Geometry: final body of the model. Coordinates: model frame, mm. Face numbers are marked on the shaded views. Round coordinates to 2 decimals unless told otherwise and drop trailing zeros. Order: outer loops, then holes, each group sorted by start corner. A loop starts at its lowest first (then second) coordinate and runs counter-clockwise, first axis right, second up. Notation, with made-up numbers: (37.25, 7.25) - (49.25, 7.25) arc R19 ccw to (49.25, 39.25) - close; hole circle Ø4 at (42.25, -40). An arc over 180 degrees is marked (long way). Put each result on its own line as item: value. Start each with the question number.
(1) Section C-C (y = -1886.5). Output: boundary loops of the cut face in (x, z), and give its area (3 significant figures).
(2) Pin query (flat end, axial travel): P1, Ø6, axis at x = -21.5, y = -366, coming from the +Z side; P2, Ø2, axis at y = -1765.5, z = 63.5, coming from the -X side; P3, Ø1, axis at y = -359, z = -63.5, coming from the -X side. Return the tip coordinate at first contact, or that it passes through.
(3) Pull-direction query (Y, two-part tool) for the marked faces 1, 2 and 3; classes: released by +Y, released by -Y, zero draft, split by the parting line, or undercut.
(4) Section B-B (z = -42.5). Output: boundary loops of the cut face in (x, y).
(5) Material intervals for L1, parallel to Z at x = -75, y = -2038.5; L2, parallel to Z at x = -75, y = 6; L3, parallel to Z at x = 0, y = -1175, sorted ascending. Write a range as [from, to].
(6) Section A-A (x = -23.5). Output: boundary loops of the cut face in (y, z).
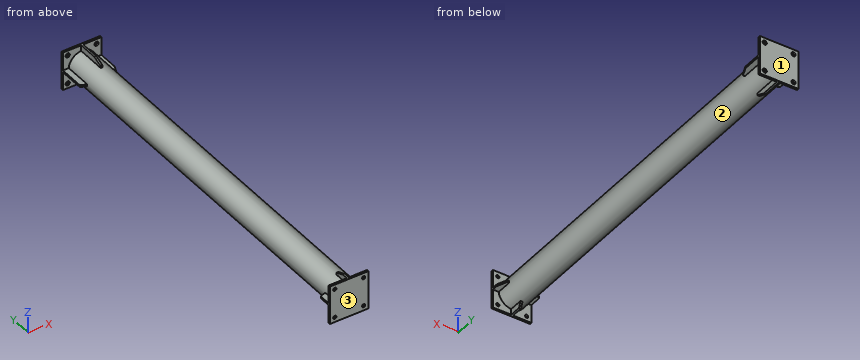
from build123d import *

# Parameters (mm, degrees)
F0_R          = 70
F0_R_2        = 65
F1_DEPTH      = 2036
F2_W          = 200
F2_H          = 200
F2_R          = 11
F3_DEPTH      = 10
F4_W          = 30.1787997812
F4_H          = 10
F4_W_2        = 10
F4_H_2        = 30.1787997812
F5_DEPTH      = 150
F6_T1_DEPTH   = 269.311363913
F6_T3_DEPTH   = 269.311363913
F6_T8_DEPTH   = 269.311363913
F6_S9_R       = 70
F6_T10_DEPTH  = 139
F8_W          = 200
F8_H          = 200
F8_R          = 8.5
F9_DEPTH      = 10
F10_W         = 10
F10_H         = 30.1787997812
F10_W_2       = 30.1787997812
F10_H_2       = 10
F11_DEPTH     = 80
F12_T1_DEPTH  = 269.311363913
F12_T3_DEPTH  = 269.311363913
F12_T8_DEPTH  = 269.311363913
F12_S9_R      = 70
F12_T10_DEPTH = 139
F12_T14_DEPTH = 269.311363913
F12_S15_R     = 70
F12_T16_DEPTH = 139


# Not quite as in the source:
# - a fillet or chamfer that OpenCascade refuses, or shapes differently, is made with other operations: its cross-section is extruded or revolved along the edge and cut away or added


with BuildPart() as f1:
    # F0 (on Front) → F1 (new body)
    with BuildSketch(Plane.XZ):
        Circle(F0_R)
        Circle(F0_R_2, mode=Mode.SUBTRACT)
    extrude(amount=F1_DEPTH)

    # F2 (on Front) → F3 (join)
    with BuildSketch(Plane.XZ):
        Rectangle(F2_W, F2_H)
        with Locations((-75, -75)):
            Circle(F2_R, mode=Mode.SUBTRACT)
        with Locations((75, -75)):
            Circle(F2_R, mode=Mode.SUBTRACT)
        with Locations((-75, 75)):
            Circle(F2_R, mode=Mode.SUBTRACT)
        with Locations((75, 75)):
            Circle(F2_R, mode=Mode.SUBTRACT)
    extrude(amount=-F3_DEPTH)

    # F4 (on Front) → F5 (join)
    with BuildSketch(Plane.XZ):
        with Locations((-84.9106001094, 0)):
            Rectangle(F4_W, F4_H)
        with Locations((0, 84.9106001094)):
            Rectangle(F4_W_2, F4_H_2)
        with Locations((84.9106001094, 0)):
            Rectangle(F4_W, F4_H)
        with Locations((0, -84.9106001094)):
            Rectangle(F4_W_2, F4_H_2)
    extrude(amount=F5_DEPTH)

    # F6: chamfer of 50 x 20 on 4 edges, made by hand

    # F6_s2 → F6_t1 (cut)
    with BuildSketch(Plane.YZ.offset(-134.6556819565)):
        Polygon((-100, 100), (-150, 80), (-150, 100), align=None)
        Polygon((-100, -100), (-150, -80), (-150, -100), align=None)
    extrude(amount=F6_T1_DEPTH, mode=Mode.SUBTRACT)

    # F6_s4 → F6_t3 (cut)
    with BuildSketch(Plane.XY.offset(-134.6556819565)):
        Polygon((100, -100), (80, -150), (100, -150), align=None)
    extrude(amount=F6_T3_DEPTH, mode=Mode.SUBTRACT)


with BuildPart() as f6_tool6:
    # F6_s7 → F6_t8 (new body)
    with BuildSketch(Plane.XY.offset(134.6556819565)):
        Polygon((-100, -130), (-50, -150), (-100, -150), align=None)
    extrude(amount=-F6_T8_DEPTH)

    # F6_s9 → F6_t10 (cut, symmetric)
    with BuildSketch(Plane.XZ.offset(140)):
        Circle(F6_S9_R)
    extrude(amount=F6_T10_DEPTH, both=True, mode=Mode.SUBTRACT)


with BuildPart() as f1_1:
    add(f1.part)

    # F6_t5: cut F6_tool6
    add(f6_tool6.part, mode=Mode.SUBTRACT)

    # F8 (on offset) → F9 (join)
    with BuildSketch(Plane.XZ.offset(2036)):
        Rectangle(F8_W, F8_H)
        with Locations((-75, -75)):
            Circle(F8_R, mode=Mode.SUBTRACT)
        with Locations((75, -75)):
            Circle(F8_R, mode=Mode.SUBTRACT)
        with Locations((-75, 75)):
            Circle(F8_R, mode=Mode.SUBTRACT)
        with Locations((75, 75)):
            Circle(F8_R, mode=Mode.SUBTRACT)
    extrude(amount=F9_DEPTH)

    # F10 (on face) → F11 (join)
    with BuildSketch(Plane(origin=(0, -2036, 0), x_dir=(-1, 0, 0), z_dir=(0, 1, 0))):
        with Locations((0, 84.9106001094)):
            Rectangle(F10_W, F10_H)
        with Locations((84.9106001094, 0)):
            Rectangle(F10_W_2, F10_H_2)
        with Locations((0, -84.9106001094)):
            Rectangle(F10_W, F10_H)
        with Locations((-84.9106001094, 0)):
            Rectangle(F10_W_2, F10_H_2)
    extrude(amount=F11_DEPTH)

    # F12: chamfer of 20 x 50 on 4 edges, made by hand

    # F12_s2 → F12_t1 (cut)
    with BuildSketch(Plane.YZ.offset(-134.6556819565)):
        Polygon((-2006, 100), (-1956, 80), (-1956, 100), align=None)
    extrude(amount=F12_T1_DEPTH, mode=Mode.SUBTRACT)

    # F12_s4 → F12_t3 (cut)
    with BuildSketch(Plane.XY.offset(-134.6556819565)):
        Polygon((100, -2006), (80, -1956), (100, -1956), align=None)
    extrude(amount=F12_T3_DEPTH, mode=Mode.SUBTRACT)


with BuildPart() as f12_tool6:
    # F12_s7 → F12_t8 (new body)
    with BuildSketch(Plane.XY.offset(-134.6556819565)):
        Polygon((-100, -1976), (-50, -1956), (-100, -1956), align=None)
    extrude(amount=F12_T8_DEPTH)

    # F12_s9 → F12_t10 (cut, symmetric)
    with BuildSketch(Plane.XZ.offset(1966)):
        Circle(F12_S9_R)
    extrude(amount=F12_T10_DEPTH, both=True, mode=Mode.SUBTRACT)


with BuildPart() as f1_2:
    add(f1_1.part)

    # F12_t5: cut F12_tool6
    add(f12_tool6.part, mode=Mode.SUBTRACT)


with BuildPart() as f12_tool12:
    # F12_s13 → F12_t14 (new body)
    with BuildSketch(Plane.YZ.offset(134.6556819565)):
        Polygon((-1976, -100), (-1956, -50), (-1956, -100), align=None)
    extrude(amount=-F12_T14_DEPTH)

    # F12_s15 → F12_t16 (cut, symmetric)
    with BuildSketch(Plane.XZ.offset(1966)):
        Circle(F12_S15_R)
    extrude(amount=F12_T16_DEPTH, both=True, mode=Mode.SUBTRACT)


with BuildPart() as f1_3:
    add(f1_2.part)

    # F12_t11: cut F12_tool12
    add(f12_tool12.part, mode=Mode.SUBTRACT)


solid = f1_3.part
Checks:
1. outline: circle Ø140 at (0, 0); hole circle Ø130 at (0, 0)
1. area: 2,120 mm²
2. P1: stops at z = 67.51
2. P2: stops at x = -31.52
2. P3: stops at x = -30.51
3. face 1: released by +Y
3. face 2: undercut
3. face 3: released by -Y
4. outline: (-100, -2046) - (100, -2046) - (100, -2036) - (55.62, -2036) - (55.62, 0) - (100, 0) - (100, 10) - (-100, 10) - (-100, 0) - (-55.62, 0) - (-55.62, -2036) - (-100, -2036) - close; hole (-49.18, -2036) - (49.18, -2036) - (49.18, 0) - (-49.18, 0) - close
5. L1: z = [-100, -83.5], [-66.5, 66.5], [83.5, 100]
5. L2: z = [-100, -86], [-64, 64], [86, 100]
5. L3: z = [-70, -65], [65, 70]
6. outline: (-2046, -100) - (-2036, -100) - (-2036, -65.94) - (0, -65.94) - (0, -100) - (10, -100) - (10, 100) - (0, 100) - (0, 65.94) - (-2036, 65.94) - (-2036, 100) - (-2046, 100) - close; hole (-2036, -60.6) - (0, -60.6) - (0, 60.6) - (-2036, 60.6) - close
